The model under review builds one solid part; all positions refer to its coordinate system, in mm. A direction names the side the tool comes from. Give positions to 0.01 mm unless a question says otherwise; leave off trailing zeros. Loops run counter-clockwise (first coordinate to the right, second up) from the corner with the lowest first, then second, coordinate; pieces in that order, holes last. Notation, with made-up numbers: M -17,-2.5 L -9,-2.5 A12 cw -9,7.5 Z; hole C -33,-3 d4. An arc over 180 degrees is marked long. Return JSON: item names as keys, results as strings.
```python
from build123d import *

# Parameters (mm, degrees)
SKETCH2_W           = 1500
SKETCH2_H           = 1500
BOSS_EXTRUDE1_DEPTH = 10
BOSS_EXTRUDE2_DEPTH = 110
BOSS_EXTRUDE3_DEPTH = 110


with BuildPart() as part:
    # Sketch2 → Boss-Extrude1 (new body)
    with BuildSketch(Plane(origin=(0, 0, 0), x_dir=(1, 0, 0), z_dir=(0, 1, 0))):
        Rectangle(SKETCH2_W, SKETCH2_H)
    extrude(amount=BOSS_EXTRUDE1_DEPTH)

    # Sketch3 → Boss-Extrude2 (add)
    with BuildSketch(Plane(origin=(0, 10, 0), x_dir=(1, 0, 0), z_dir=(0, 1, 0))):
        with BuildLine():
            ThreePointArc((750, -600), (-204.594154602, -204.594154602), (-600, 750))
            Line((-600, 750), (-620, 750))
            ThreePointArc((-620, 750), (-218.736290226, -218.736290226), (750, -620))
            Line((750, -620), (750, -600))
        make_face()
        with BuildLine():
            Line((620, 750), (600, 750))
            ThreePointArc((600, 750), (643.933982822, 643.933982822), (750, 600))
            Line((750, 600), (750, 620))
            ThreePointArc((750, 620), (658.076118446, 658.076118446), (620, 750))
        make_face()
    extrude(amount=BOSS_EXTRUDE2_DEPTH)

    # Sketch4 → Boss-Extrude3 (add)
    with BuildSketch(Plane(origin=(0, 10, 0), x_dir=(1, 0, 0), z_dir=(0, 1, 0))):
        Polygon((-197.52308679, -211.665222414), (-91.457069612, -105.599205236), (-105.599205236, -91.457069612), (-211.665222414, -197.52308679), align=None)
    extrude(amount=BOSS_EXTRUDE3_DEPTH)


solid = part.part
```
1) Insertion check: pin 1 (2 mm diameter, centred on x = -77.5, y = 38.5, fed in from -Z); pin 2 (1.5 mm diameter, centred on x = -85.5, y = 48, fed in from -Z); pin 3 (5 mm diameter, centred on y = 13, z = -389, fed in from -X). Each pin has a flat end and moves straight along its axis. Give the tip position at first contact, or say it passes through.
From the geometry:
{"pin 1": "z = 315.87", "pin 2": "z = 309.8", "pin 3": "x = -572.26"}
2) The part is to be moulded in two halves that separate along X. For faces 4 (the face through (-496.335, 64.23, -231.205)), 5 (the face through (-229.329, 64.23, 208.026)), 6 (the face through (652, 120, -659)), 7 (the face through (-145.22, 64.23, 159.36)), say which applies: released by +X, released by -X, zero draft, split by the parting line, or undercut.
From the geometry:
{"face 4": "undercut", "face 5": "released by -X", "face 6": "zero draft", "face 7": "released by +X"}
3) Consider section B-B on z = -225. Write out the cut boundary in (x, y), then the cut area to 3 significant figures.
From the geometry:
{"outline": "M -750,0 L 750,0 L 750,10 L -493.73,10 L -493.73,120 L -515.41,120 L -515.41,10 L -750,10 Z", "area": "17,400 mm²"}
4) Consider section C-C on x = -360.5. Write out the cut boundary in (y, z).
From the geometry:
{"outline": "M 0,-750 L 10,-750 L 10,17.65 L 120,17.65 L 120,52.3 L 10,52.3 L 10,750 L 0,750 Z"}
5) Consider section A-A on y = 37. Write out the cut boundary in (x, z), then the cut area to 3 significant figures.
From the geometry:
{"outline": "M -620,-750 L -600,-750 A1350 cw -211.64,197.5 L -105.6,91.46 L -91.46,105.6 L -197.5,211.64 A1350 cw 750,600 L 750,620 A1370 ccw Z; M 600,-750 L 620,-750 A130 cw 750,-620 L 750,-600 A150 ccw Z", "area": "50,100 mm²"}
6) Wall thickness on L1, parallel to Y at x = -23, z = 270; L2, parallel to X at y = 113, z = -675; L3, parallel to X at y = 90, z = -640: over which ranges is each line inside the solid? List them lowest first. Write a range as from..to.
From the geometry:
{"L1": "0..10", "L2": "-617.95..-597.92, 620.1..643.82", "L3": "-615.58..-595.51, 648.02..680.72"}
7) Tool access review of faces 1 (the face through (-157.877, 64.23, 143.735)), 2 (the face through (216, 10, -234)), 3 (the face through (-337, 10, 274)): name each direction out of +Z, -Z, +X, -X, +Y, -Y from which nothing blocks a thin tool from reaching the whole face with its end or side.
From the geometry:
{"face 1": "-Z, +Y", "face 2": "+Y", "face 3": "+Z, -X, +Y"}
